Input: dimensioned drawing with shaded views. Units: mm. Origin: part minimum x, y, z. Round coordinates to 2 decimals unless told otherwise and drop trailing zeros. Loops run counter-clockwise (first coordinate to the right, second up) from the corner with the lowest first, then second, coordinate; pieces in that order, holes last. Notation, with made-up numbers: M 11,51.5 L 28,51.5 A23 cw 28,60.5 Z; hole C 87,88.25 d6. An arc over 180 degrees is marked long. Answer as a JSON object with one key per item and string values.
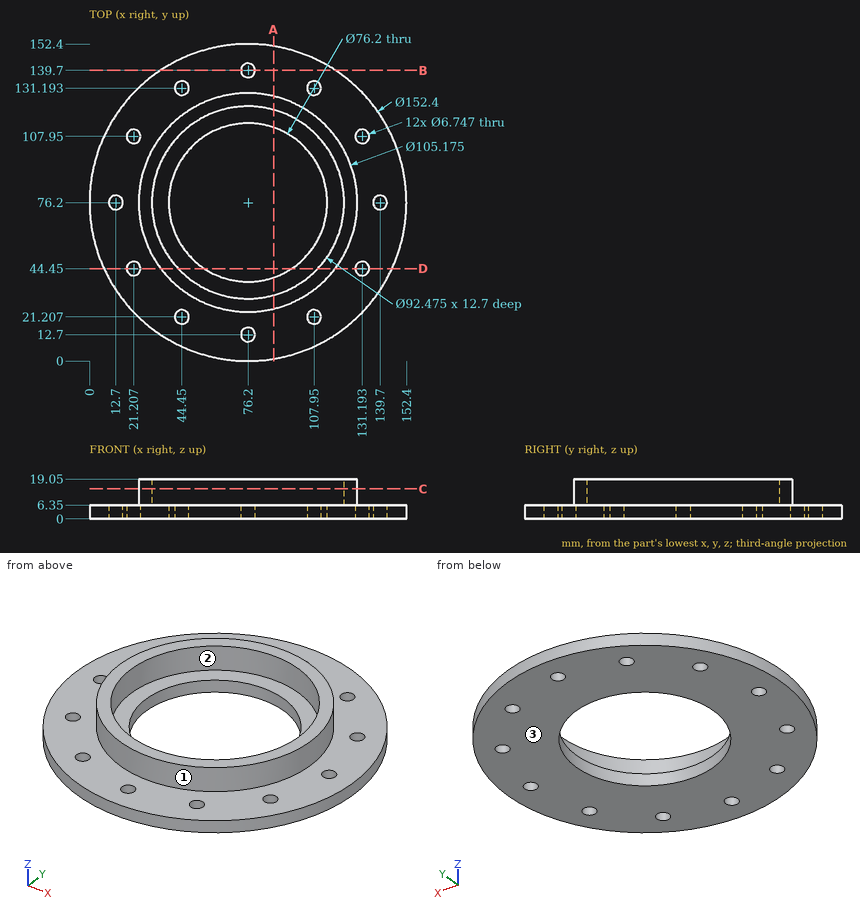
Item 1: Section C-C on z = 14.25. Return the cut outline in (x, y) (1 decimal).
Answer sheet:
{"outline": "C 76.2,76.2 d105.2; hole C 76.2,76.2 d92.5"}
Item 2: Line query: probe 1 along Y at (x, z) = (128.5, 4.25) (1 decimal); probe 2 along Y at (x, z) = (44.45, 2) (1 decimal); probe 3 along Z at (x, y) = (26.5, 34). Output: solid intervals per line, ascending. Write a range as from..to.
Answer sheet:
{"probe 1": "y = 20.8..42.4, 46.5..105.9, 110..131.6", "probe 2": "y = 6.9..17.8, 24.6..55.1, 97.3..127.8, 134.6..145.5", "probe 3": "z = 0..6.35"}
Item 3: Pull-direction query (X, two-part tool) for the marked faces 1, 2 and 3; classes: pulls with the +X half, pulls with the -X half, needs draft (parallel to the pull), parting line crosses it, or undercut.
Answer sheet:
{"face 1": "parting line crosses it", "face 2": "undercut", "face 3": "needs draft"}
Item 4: Section B-B on y = 139.7. Return the cut outline in (x, z).
Answer sheet:
{"outline": "M 34.08,0 L 72.83,0 L 72.83,6.35 L 34.08,6.35 Z; M 79.57,0 L 118.32,0 L 118.32,6.35 L 79.57,6.35 Z"}
Item 5: Section A-A on x = 88.5. Return the cut outline in (y, z).
Answer sheet:
{"outline": "M 1,0 L 40.14,0 L 40.14,6.35 L 31.63,6.35 L 31.63,19.05 L 25.07,19.05 L 25.07,6.35 L 1,6.35 Z; M 112.26,0 L 151.4,0 L 151.4,6.35 L 127.33,6.35 L 127.33,19.05 L 120.77,19.05 L 120.77,6.35 L 112.26,6.35 Z"}
Item 6: Contact query for flat-ended pins moving along their axis: pin 1 Ø6 at (x, y) = (131.19, 44.45) entering from +Z; pin 2 Ø5 at (x, y) = (68.5, 34.5) entering from +Z; pin 3 Ø1 at (y, z) = (98, 3) entering from +X; pin 4 Ø4 at (x, z) = (47, 11) entering from -Y. Output: stop coordinate, or through.
Answer sheet:
{"pin 1": "passes through", "pin 2": "stops at z = 6.35", "pin 3": "stops at x = 149.36", "pin 4": "stops at y = 31.19"}
Item 7: Section D-D on y = 44.45. Return the cut outline in (x, z).
Answer sheet:
{"outline": "M 6.93,0 L 17.83,0 L 17.83,6.35 L 6.93,6.35 Z; M 24.58,0 L 55.14,0 L 55.14,6.35 L 42.59,6.35 L 42.59,19.05 L 34.28,19.05 L 34.28,6.35 L 24.58,6.35 Z; M 97.26,0 L 127.82,0 L 127.82,6.35 L 118.12,6.35 L 118.12,19.05 L 109.81,19.05 L 109.81,6.35 L 97.26,6.35 Z; M 134.57,0 L 145.47,0 L 145.47,6.35 L 134.57,6.35 Z"}
